from build123d import *

# Parameters (mm, degrees)
BOSS_EXTRUDE1_DEPTH     = 12
CUT_EXTRUDE1_DEPTH      = 26.768197453
CUT_EXTRUDE1_DEPTH_BACK = 26.768197453
SKETCH2_R               = 3.15


with BuildPart() as part:
    # Sketch1 → Boss-Extrude1 (new body)
    with BuildSketch(Plane.XY):
        with BuildLine():
            Line((0, 6), (22, 6))
            Line((22, 6), (22, 2.552710574))
            Line((22, 2.552710574), (2.091331807, 2.552710574))
            ThreePointArc((2.091331807, 2.552710574), (-3.3, 0), (2.091331807, -2.552710574))
            Line((2.091331807, -2.552710574), (22, -2.552710574))
            Line((22, -2.552710574), (22, -6))
            Line((22, -6), (0, -6))
            ThreePointArc((0, -6), (-6, 0), (0, 6))
        make_face()
    extrude(amount=BOSS_EXTRUDE1_DEPTH)

    # Sketch2 → Cut-Extrude1 (cut, two sides: drawn at the far end of the back side and taken through both)
    with BuildSketch(Plane(origin=(0, 0, 0), x_dir=(1, 0, 0), z_dir=(0, 1, 0)).offset(-CUT_EXTRUDE1_DEPTH_BACK)):
        with Locations(Location((16, -6, 0), (0, 0, 270))):
            Circle(SKETCH2_R)
    extrude(amount=CUT_EXTRUDE1_DEPTH + CUT_EXTRUDE1_DEPTH_BACK, mode=Mode.SUBTRACT)


solid = part.part
Input: part model. Units: mm. Frame: model coordinates. A direction names the side the tool comes from. Give positions to 0.01 mm unless a question says otherwise; leave off trailing zeros. Order: outer loops, then holes, each group sorted by start corner. A loop starts at its lowest first (then second) coordinate and runs counter-clockwise, first axis right, second up. Notation, with made-up numbers: M 46.5,-32.75 L 88.5,-32.75 A27 cw 88.5,-9.75 Z; hole C -1.75,72.25 d7. An arc over 180 degrees is marked long. Answer as a JSON object with one key per item and string values.
1. Cut plane B-B, the plane z = 6. Output: boundary loops of the cut face in (x, y), and give its area (3 significant figures).
Result sheet:
{"outline": "M 0,-6 L 12.85,-6 L 12.85,-2.55 L 2.09,-2.55 A3.3 cw long 2.09,2.55 L 12.85,2.55 L 12.85,6 L 0,6 A6 ccw Z; M 19.15,-6 L 22,-6 L 22,-2.55 L 19.15,-2.55 Z; M 19.15,2.55 L 22,2.55 L 22,6 L 19.15,6 Z", "area": "146 mm²"}
2. Cut plane D-D, the plane y = 3.75. Output: boundary loops of the cut face in (x, z).
Result sheet:
{"outline": "M -4.68,0 L 22,0 L 22,12 L -4.68,12 Z; hole C 16,6 d6.3"}
3. Cut plane C-C, the plane x = 8. Output: boundary loops of the cut face in (y, z), and give its area (3 significant figures).
Result sheet:
{"outline": "M -6,0 L -2.55,0 L -2.55,12 L -6,12 Z; M 2.55,0 L 6,0 L 6,12 L 2.55,12 Z", "area": "82.7 mm²"}
4. Cut plane A-A, the plane x = 16. Output: boundary loops of the cut face in (y, z).
Result sheet:
{"outline": "M -6,0 L -2.55,0 L -2.55,2.85 L -6,2.85 Z; M -6,9.15 L -2.55,9.15 L -2.55,12 L -6,12 Z; M 2.55,0 L 6,0 L 6,2.85 L 2.55,2.85 Z; M 2.55,9.15 L 6,9.15 L 6,12 L 2.55,12 Z"}
5. Reachability of faces 4 (the flat face through (12, 2.553, 6)), 5 (the cylindrical face through (14.79, 4.25, 8.91)) from +Z, -Z, +X, -X, +Y, -Y: full face, straight path, thin tool, end or side. Return the list, or none.
Result sheet:
{"face 4": "+Z, -Z, +X", "face 5": "+Y, -Y"}
6. Pull-direction query (Z, two-part tool) for faces 1 (the flat face through (12, -2.553, 6)), 2 (the cylindrical face through (14.79, -4.3, 8.91)), 3 (the flat face through (8, 3, 0)); classes: +Z half, -Z half, draft (parallel to the pull), parting line (faces both ways), or undercut.
Result sheet:
{"face 1": "draft", "face 2": "undercut", "face 3": "-Z half"}
7. First-contact query: P1, Ø3, axis at y = -3, z = 3.5, coming from the -X side; P2, Ø6, axis at y = 4, z = 3.5, coming from the -X side. Flat tips, straight axial feed; report the tip coordinate or a pass-through.
Result sheet:
{"P1": "x = -5.81", "P2": "x = -5.92"}
8. Ray query, line 1 (Y direction, x = 6.75, z = 9.25); line 2 (Y direction, x = 0, z = 7.5); line 3 (Z direction, x = 16, y = -3.95). Return the intervals inside material, ascending. Write a range as [from, to].
Result sheet:
{"line 1": "[-6, -2.55], [2.55, 6]", "line 2": "[-6, -3.3], [3.3, 6]", "line 3": "[0, 2.85], [9.15, 12]"}
